Model file for the job. Use its own axes, mm. Face numbers are marked on the shaded views. Give positions to 0.01 mm unless a question says otherwise; leave off trailing zeros. Loops run counter-clockwise (first coordinate to the right, second up) from the corner with the lowest first, then second, coordinate; pieces in that order, holes last. Notation, with made-up numbers: M 56.25,46.5 L 68.25,46.5 A30 cw 68.25,74.5 Z; hole C 74.5,-39 d5. An arc over 180 degrees is marked long. Use CSV: the item, a comma, the result in double quotes. Start each with the question number.
(1) Two-plate mould, pull along X, no slides. Class the marked faces 1, 2 and 3: pulls with the +X half, pulls with the -X half, needs draft (parallel to the pull), parting line crosses it, or undercut.
(2) Slice it at D-D on x = 7.25. State how many separate pieces and enclosed holes the cut face has, and give its area (3 significant figures).
(3) Flat gauge pins, fed straight in: P1, Ø1.3, axis at x = 6.5, z = 0, coming from the +Y side; P2, Ø1, axis at x = -2, y = -6.5, coming from the -Z side; P3, Ø0.6, axis at x = 3, y = -7, coming from the +Z side. Where does each tip first touch, or does it go through?
(4) Slice it at A-A on z = -4.5. List the corners of the cut face in (x, y), and give its area (3 significant figures).
(5) Slice it at C-C on z = 3.75. List the corners of the cut face in (x, y), and give its area (3 significant figures).
(6) Slice it at B-B on y = 0. List the corners of the cut face in (x, z).
(7) Wall check: line 1 along Y through (x, z) = (0, 6.15); line 2 along Y through (x, z) = (-6, 2); line 3 along X through (y, z) = (-4.75, 2). Give the ranges that are in metal, low to high. Write a range as from..to.
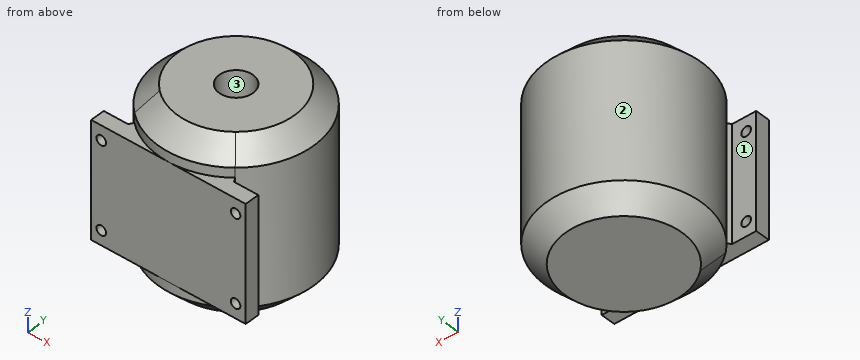
Autodesk Inventor part; units mm, degrees
ref_plane "YZ Plane" through (0, 0, 0) normal (1, 0, 0) x (0, 1, 0)
ref_plane "XZ Plane" through (0, 0, 0) normal (0, 1, 0) x (-1, 0, 0)
ref_plane "XY Plane" through (0, 0, 0) normal (0, 0, 1) x (1, 0, 0)
sketch "Sketch1" plane through (0, 0, 0) normal (0, 0, 1) x (1, 0, 0)
  arc A0 (5.2535, -6.0994) -> (-5.2535, -6.0994) centre (0, 0) ccw
  line L0 (0, 0) -> (0, -8.05) construction
  line L1 (0, -8.05) -> (8.05, -8.05)
  line L2 (8.05, -8.05) -> (8.05, -6.55)
  line L3 (8.05, -6.55) -> (5.5137, -6.55)
  line L4 (0, 0) -> (4.025, -6.9715) construction
  line L5 (5.5137, -6.55) -> (5.2535, -6.0994)
  line L6 (0, 0) -> (8.05, 0) construction
  line L7 (0, -8.05) -> (-8.05, -8.05)
  line L8 (-8.05, -8.05) -> (-8.05, -6.55)
  line L9 (-8.05, -6.55) -> (-5.5137, -6.55)
  line L10 (-5.5137, -6.55) -> (-5.2535, -6.0994)
  dimension "d0" = 16.1
  dimension "d1" = 30
  dimension "d2" = 1.5
  dimension "d3" = 1.5
extrude "Extrusion1" add sketch "Sketch1" along normal mid plane 12
sketch "Sketch2" plane through (0, 0, 0) normal (0, 0, 1) x (1, 0, 0)
  arc A0 (5.2535, -6.0994) -> (-5.2535, -6.0994) centre (0, 0) ccw
  circle A1 centre (0, 0) radius 8.05
  point P0 (4.8598, -6.4175)
extrude "Extrusion2" add sketch "Sketch2" along normal mid plane 18
chamfer "Chamfer1" distance 2 angle 45 2 edges at (-8.05, 0, 9) (-8.05, 0, -9)
sketch "Sketch3" plane through (0, 0, 9) normal (0, 0, 1) x (1, 0, 0)
  circle A0 centre (0, 0) radius 6.05
  circle A1 centre (0, 0) radius 1.75
  dimension "d11" = 3.5
extrude "Extrusion3" cut sketch "Sketch3" against normal blind 4 contours A1
sketch "Sketch4" plane through (-8.05, -8.05, 6) normal (0, -1, 0) x (1, 0, 0)
  line L0 (0, -12) -> (0, 0)
  line L1 (16.1, -12) -> (16.1, 0)
  line L2 (16.1, 0) -> (8.05, 0)
  line L3 (8.05, 0) -> (8.05, -12) construction
  line L4 (0, -6) -> (16.1, -6) construction
  line L5 (1.05, -1.5) -> (15.05, -1.5) construction
  line L6 (15.05, -1.5) -> (15.05, -10.5) construction
  line L7 (15.05, -10.5) -> (1.05, -10.5) construction
  line L8 (1.05, -10.5) -> (1.05, -1.5) construction
  circle A0 centre (1.05, -1.5) radius 0.5
  circle A1 centre (15.05, -1.5) radius 0.5
  circle A2 centre (1.05, -10.5) radius 0.5
  circle A3 centre (15.05, -10.5) radius 0.5
  dimension "d14" = 9
  dimension "d15" = 4.5
  dimension "d16" = 14
  dimension "d17" = 7
  dimension "d18" = 1
extrude "Extrusion4" cut sketch "Sketch4" against normal up to surface (1.5 mm away)
properties part number "Motor"
Reply:
1,face 1,"needs draft"
1,face 2,"parting line crosses it"
1,face 3,"undercut"
2,separate pieces,"4"
2,enclosed holes,"0"
2,area,"121 mm^2"
3,P1,"stops at y = 5.53"
3,P2,"stops at z = -8.75"
3,P3,"stops at z = 7.73"
4,outline,"M -8.05,-8.05 L -7.5,-8.05 L -7.5,-6.55 L -8.05,-6.55 Z; M -6.5,-8.05 L 6.5,-8.05 L 6.5,-6.55 L 5.51,-6.55 L 5.25,-6.1 A8.05 ccw long -5.25,-6.1 L -5.51,-6.55 L -6.5,-6.55 Z; M 7.5,-8.05 L 8.05,-8.05 L 8.05,-6.55 L 7.5,-6.55 Z"
4,area,"216 mm^2"
5,outline,"M -8.05,-8.05 L 8.05,-8.05 L 8.05,-6.55 L 5.51,-6.55 L 5.25,-6.1 A8.05 ccw long -5.25,-6.1 L -5.51,-6.55 L -8.05,-6.55 Z"
5,area,"219 mm^2"
6,outline,"M -8.05,-7 L -6.05,-9 L 6.05,-9 L 8.05,-7 L 8.05,7 L 6.05,9 L 1.75,9 L 1.75,5 L -1.75,5 L -1.75,9 L -6.05,9 L -8.05,7 Z"
7,line 1,"y = -8.05..-1.75, 1.75..8.05"
7,line 2,"y = -8.05..-6.55, -5.37..5.37"
7,line 3,"x = -6.5..6.5"
